For this review, take the finished solid that the model builds, in its own axes (mm). Give positions to 0.01 mm unless a question says otherwise; leave off trailing zeros. Order: outer loops, then holes, each group sorted by start corner. A loop starts at its lowest first (then second) coordinate and runs counter-clockwise, first axis right, second up. Notation, with made-up numbers: (8, 50.5) -> (42, 50.5) arc R17 ccw to (42, 56.5) -> close; hole circle Ø8 at (-12, 77). An arc over 180 degrees is marked (long way). Return JSON: item names as keys, results as strings. Group by question number.
1) Add section B-B (x = 13). Give the boundary of the cut face in (y, z), then the cut area to 3 significant figures.
2) To check wall thickness, follow line 1 along Z through (x, y) = (-4, -55); line 2 along X through (y, z) = (-22, -0.25). State the ranges of each line that lie inside material, in increasing order.
3) Add section A-A (y = -61). Give the boundary of the cut face in (x, z).
4) Insertion check: P1, Ø5, axis at x = 11, y = -57, coming from the -Z side. The pin has a flat end and moves straight along its axis. Give the tip position at first contact, or say it passes through.
from build123d import *

# Parameters (mm, degrees)
SKETCH_1_W      = 31.172738554
SKETCH_1_H      = 53.896192989
EXTRUDE_1_DEPTH = 10
SKETCH_2_W      = 10
SKETCH_2_H      = 5
EXTRUDE_3_DEPTH = 1.2
FILLET_1_R      = 1
FILLET_2_R      = 1


with BuildPart() as part:
    # 草圖1 → 填料-伸長1 (new body)
    with BuildSketch(Plane.XY):
        with Locations((0, -43.60381631)):
            Rectangle(SKETCH_1_W, SKETCH_1_H)
    extrude(amount=EXTRUDE_1_DEPTH)

    # 草圖2 → 填料-伸長3 (add)
    with BuildSketch(Plane.XY):
        with Locations((0, -20.178917106)):
            Rectangle(SKETCH_2_W, SKETCH_2_H)
    extrude(amount=-EXTRUDE_3_DEPTH)

    # 圓角1
    fillet_1_edges = [part.edges().sort_by_distance(p)[0] for p in [
        (-5, -20.178917106, -1.2),
        (0, -17.678917106, -1.2),
        (5, -20.178917106, -1.2),
        (0, -22.678917106, -1.2),
    ]]
    fillet(fillet_1_edges, radius=FILLET_1_R)

    # 圓角2
    fillet_2_edges = [part.edges().sort_by_distance(p)[0] for p in [
        (-15.586369277, -43.60381631, 10),
        (0, -70.551912804, 10),
        (15.586369277, -43.60381631, 10),
        (0, -70.551912804, 0),
        (-15.586369277, -43.60381631, 0),
        (0, -16.655719815, 0),
        (15.586369277, -43.60381631, 0),
        (15.586369277, -70.551912804, 5),
        (-15.586369277, -70.551912804, 5),
        (-15.586369277, -16.655719815, 5),
        (15.586369277, -16.655719815, 5),
        (0, -16.655719815, 10),
    ]]
    fillet(fillet_2_edges, radius=FILLET_2_R)


solid = part.part
Evaluation:
{
 "1": {"outline": "(-70.55, 1) arc R1 ccw to (-69.55, 0) -> (-17.66, 0) arc R1 ccw to (-16.66, 1) -> (-16.66, 9) arc R1 ccw to (-17.66, 10) -> (-69.55, 10) arc R1 ccw to (-70.55, 9) -> close", "area": "538 mm^2"},
 "2": {"line 1": "0 to 10", "line 2": "-5 to 5"},
 "3": {"outline": "(-15.59, 1) arc R1 ccw to (-14.59, 0) -> (14.59, 0) arc R1 ccw to (15.59, 1) -> (15.59, 9) arc R1 ccw to (14.59, 10) -> (-14.59, 10) arc R1 ccw to (-15.59, 9) -> close"},
 "4": {"P1": "z = 0"}
}
